```python
from build123d import *

# Parameters (mm, degrees)
F0_R     = 38.1
F0_W     = 12.7
F0_H     = 25.4
F1_DEPTH = 50.8


with BuildPart() as f1:
    # F0 (on Top) → F1 (new body, symmetric)
    with BuildSketch(Plane.XY):
        with BuildLine():
            Line((82.55, 22.225), (47.625, 22.225))
            ThreePointArc((47.625, 22.225), (45.991476, 22.67746), (44.823529, 23.905882))
            ThreePointArc((44.823529, 23.905882), (-50.8, 0), (44.823529, -23.905882))
            ThreePointArc((44.823529, -23.905882), (45.991476, -22.67746), (47.625, -22.225))
            Line((47.625, -22.225), (82.55, -22.225))
            ThreePointArc((82.55, -22.225), (84.795064, -21.295064), (85.725, -19.05))
            Line((85.725, -19.05), (85.725, 19.05))
            ThreePointArc((85.725, 19.05), (84.795064, 21.295064), (82.55, 22.225))
        make_face()
        Circle(F0_R, mode=Mode.SUBTRACT)
        with Locations((66.675, 0)):
            Rectangle(F0_W, F0_H, mode=Mode.SUBTRACT)
    extrude(amount=F1_DEPTH, both=True)


solid = f1.part
```
Work out the finished part from the listing and answer in its coordinate system (mm). A direction names the side the tool comes from. Coordinates: 2 decimals unless noted, no trailing zeros. Write each loop counter-clockwise with the first axis right and the second up, starting at its lowest first coordinate (ties: lowest second). Pieces come first, ordered by that corner, then holes. Notation, with made-up numbers: (56.5, -23) - (69.5, -23) arc R18 ccw to (69.5, 11) - close; hole circle Ø4 at (1.25, -12). An arc over 180 degrees is marked (long way). Answer as a JSON object with one key per item and string values.
Q1. Given pin 1 Ø6 at (x, z) = (45.5, -40) entering from -Y; pin 2 Ø7.5 at (y, z) = (-1.5, -11.5) entering from -X; pin 3 Ø6 at (x, z) = (-11.5, -36) entering from -Y, each flat-ended and moving along its own axis, determine where each tip first touches the part or whether it passes through.
Results list:
{"pin 1": "stops at y = -27.83", "pin 2": "stops at x = -50.8", "pin 3": "stops at y = -50.08"}
Q2. Find section C-C (z = -12). Write down the section's boundary in (x, y) (3 decimals), plus the area to 3 significant figures.
Results list:
{"outline": "(44.824, -23.906) arc R3.175 cw to (47.625, -22.225) - (82.55, -22.225) arc R3.175 ccw to (85.725, -19.05) - (85.725, 19.05) arc R3.175 ccw to (82.55, 22.225) - (47.625, 22.225) arc R3.175 cw to (44.824, 23.906) arc R50.8 ccw (long way) to start; hole circle Ø76.2 at (0, 0); hole (60.325, -12.7) - (73.025, -12.7) - (73.025, 12.7) - (60.325, 12.7) - close", "area": "4,850 mm^2"}
Q3. Find section A-A (y = 0). Write down the section's boundary in (x, z) (3 decimals), plus the area to 3 significant figures.
Results list:
{"outline": "(-50.8, -50.8) - (-38.1, -50.8) - (-38.1, 50.8) - (-50.8, 50.8) - close; (38.1, -50.8) - (60.325, -50.8) - (60.325, 50.8) - (38.1, 50.8) - close; (73.025, -50.8) - (85.725, -50.8) - (85.725, 50.8) - (73.025, 50.8) - close", "area": "4,840 mm^2"}
Q4. Find section D-D (y = 35). Write down the section's boundary in (x, z), plus the area to 3 significant figures.
Results list:
{"outline": "(-36.82, -50.8) - (-15.05, -50.8) - (-15.05, 50.8) - (-36.82, 50.8) - close; (15.05, -50.8) - (36.82, -50.8) - (36.82, 50.8) - (15.05, 50.8) - close", "area": "4,420 mm^2"}
Q5. Find section B-B (x = 0). Write down the section's boundary in (y, z).
Results list:
{"outline": "(-50.8, -50.8) - (-38.1, -50.8) - (-38.1, 50.8) - (-50.8, 50.8) - close; (38.1, -50.8) - (50.8, -50.8) - (50.8, 50.8) - (38.1, 50.8) - close"}
Q6. For a pull along Y with two mould halves and no side action, classify faces 1 (the flat face through (85.725, 0, 1)), 2 (the cylindrical face through (-50.765, 1.885, 0.711)), 3 (the flat face through (67, -12.7, 1)) as pulls with the +Y half, pulls with the -Y half, needs draft (parallel to the pull), parting line crosses it, or undercut.
Results list:
{"face 1": "needs draft", "face 2": "parting line crosses it", "face 3": "undercut"}
Q7. Consider L1, parallel to Y at x = 0, z = -17; L2, parallel to X at y = 0.5, z = 5 (3 decimals); L3, parallel to X at y = -8.5, z = 34.5 (3 decimals). Determine where each line is inside the solid, lowest interval first. Write a range as from..to.
Results list:
{"L1": "y = -50.8..-38.1, 38.1..50.8", "L2": "x = -50.798..-38.097, 38.097..60.325, 73.025..85.725", "L3": "x = -50.084..-37.14, 37.14..60.325, 73.025..85.725"}
Q8. Which of the six approach directions +Z, -Z, +X, -X, +Y, -Y give full straight-line access (tool end or side, diameter ignored) to faces 4 (the flat face through (60.325, 0, -1)), 5 (the flat face through (37, -11, 50.8)), 6 (the flat face through (65, 22.225, 1)), 7 (the flat face through (65, -22.225, 1))?
Results list:
{"face 4": "+Z, -Z", "face 5": "+Z, +X, -X, +Y, -Y", "face 6": "+Z, -Z, +X, +Y", "face 7": "+Z, -Z, +X, -Y"}
